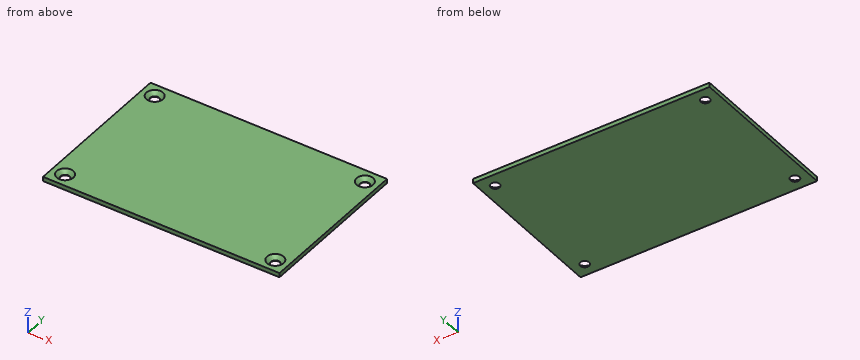
from build123d import *

# Parameters (mm, degrees)
SKETCH1_W                                           = 90
SKETCH1_H                                           = 60
BOSS_EXTRUDE1_DEPTH                                 = 1.666
CSK_FOR_M3_COUNTERSUNK_FLAT_HEAD_SCREW1_D           = 3.4
CSK_FOR_M3_COUNTERSUNK_FLAT_HEAD_SCREW1_DEPTH       = 30
CSK_FOR_M3_COUNTERSUNK_FLAT_HEAD_SCREW1_CSINK_D     = 6.3
CSK_FOR_M3_COUNTERSUNK_FLAT_HEAD_SCREW1_CSINK_ANGLE = 90
CSK_FOR_M3_COUNTERSUNK_FLAT_HEAD_SCREW1_TIP         = 1.021463052


with BuildPart() as part:
    # Sketch1 → Boss-Extrude1 (new body)
    with BuildSketch(Plane.XY):
        with Locations((45, 30)):
            Rectangle(SKETCH1_W, SKETCH1_H)
    extrude(amount=BOSS_EXTRUDE1_DEPTH)

    # CSK for M3 Countersunk Flat Head Screw1
    with Locations(Plane.XY.offset(1.666)):
        with Locations((5, 55), (5, 5), (85, 5), (85, 55)):
            CounterSinkHole(CSK_FOR_M3_COUNTERSUNK_FLAT_HEAD_SCREW1_D / 2, CSK_FOR_M3_COUNTERSUNK_FLAT_HEAD_SCREW1_CSINK_D / 2, depth=CSK_FOR_M3_COUNTERSUNK_FLAT_HEAD_SCREW1_DEPTH, counter_sink_angle=CSK_FOR_M3_COUNTERSUNK_FLAT_HEAD_SCREW1_CSINK_ANGLE)
            with Locations((0, 0, -(CSK_FOR_M3_COUNTERSUNK_FLAT_HEAD_SCREW1_DEPTH + CSK_FOR_M3_COUNTERSUNK_FLAT_HEAD_SCREW1_TIP / 2))):  # 118° drill point
                Cone(0, CSK_FOR_M3_COUNTERSUNK_FLAT_HEAD_SCREW1_D / 2, CSK_FOR_M3_COUNTERSUNK_FLAT_HEAD_SCREW1_TIP, mode=Mode.SUBTRACT)


solid = part.part
The listing builds one solid part. Answer for the finished solid, in the listing's coordinates (mm). Give positions to 0.01 mm unless a question says otherwise; leave off trailing zeros. Write each loop counter-clockwise with the first axis right and the second up, starting at its lowest first coordinate (ties: lowest second). Pieces come first, ordered by that corner, then holes. Notation, with made-up numbers: (87.25, -17.75) - (99.25, -17.75) arc R3 ccw to (99.25, -12.75) - close; hole circle Ø4 at (36, -35.75). An arc over 180 degrees is marked (long way). One line per question, with ' | ' between items. Start each with the question number.
1. Straight lines are drawn through the part: line 1 (X direction, y = 55, z = 0.15); line 2 (Y direction, x = 85, z = 0.15); line 3 (X direction, y = 4.5, z = 0.7). For each, find the intervals that lie inside material, in ascending order.
2. Section B-B, the plane x = 85 is taken. Determine the outline of the cut face in (y, z).
3. Section C-C, the plane z = 1.4 is taken. Determine the outline of the cut face in (x, y), then the cut area to 3 significant figures.
4. Given P1, Ø4.5, axis at x = 85, y = 5, coming from the +Z side, flat-ended and moving along its own axis, determine where the tip first touches the part or whether it passes through.
5. Section A-A, the plane y = 55 is taken. Determine the outline of the cut face in (x, z).
Result:
1) line 1: x = 0 to 3.3, 6.7 to 83.3, 86.7 to 90 | line 2: y = 0 to 3.3, 6.7 to 53.3, 56.7 to 60 | line 3: x = 0 to 2.87, 7.13 to 82.87, 87.13 to 90
2) outline: (0, 0) - (3.3, 0) - (3.3, 0.22) - (1.85, 1.67) - (0, 1.67) - close; (6.7, 0) - (53.3, 0) - (53.3, 0.22) - (51.85, 1.67) - (8.15, 1.67) - (6.7, 0.22) - close; (56.7, 0) - (60, 0) - (60, 1.67) - (58.15, 1.67) - (56.7, 0.22) - close
3) outline: (0, 0) - (90, 0) - (90, 60) - (0, 60) - close; hole circle Ø5.77 at (5, 5); hole circle Ø5.77 at (5, 55); hole circle Ø5.77 at (85, 5); hole circle Ø5.77 at (85, 55) | area: 5,300 mm2
4) P1: stops at z = 0.77
5) outline: (0, 0) - (3.3, 0) - (3.3, 0.22) - (1.85, 1.67) - (0, 1.67) - close; (6.7, 0) - (83.3, 0) - (83.3, 0.22) - (81.85, 1.67) - (8.15, 1.67) - (6.7, 0.22) - close; (86.7, 0) - (90, 0) - (90, 1.67) - (88.15, 1.67) - (86.7, 0.22) - close
